```python
from build123d import *

# Parameters (mm, degrees)
F1_DEPTH = 5
F3_DEPTH = 2
F4_R     = 3.5
F5_DEPTH = 5
F6_R     = 2
F7_DEPTH = 5000


with BuildPart() as f1:
    # F0 (on Front) → F1 (new body)
    with BuildSketch(Plane.XZ):
        with BuildLine():
            Line((19.9153833091, -4.2498749681), (11.3317733631, 0))
            Line((11.3317733631, 0), (9.8158549517, -3.3205298241))
            Line((9.8158549517, -3.3205298241), (12.4476579949, -2.8994414024))
            Line((12.4476579949, -2.8994414024), (16.0058550537, -4.4364142232))
            add(Edge.make_bspline(
                [(16.0058550537, -4.4364142232), (20.2167406678, -7.2366520762), (14.6583728492, -14.2898829654), (8.973678574, -6.310257595)],
                knots=[0, 0, 0, 0, 7.2775541924, 7.2775541924, 7.2775541924, 7.2775541924], degree=3))
            Line((8.973678574, -6.310257595), (7.3524885811, -9.7631821409))
            Line((7.3524885811, -9.7631821409), (6.3418764621, -14.3951550126))
            Line((6.3418764621, -14.3951550126), (6.1102770269, -19.4692704827))
            Line((6.1102770269, -19.4692704827), (8.973678574, -17.8059712052))
            Line((8.973678574, -17.8059712052), (12.5318756327, -18.0796794593))
            Line((12.5318756327, -18.0796794593), (14.805752784, -19.9956316501))
            Line((14.805752784, -19.9956316501), (15.7110933214, -23.7643718719))
            Line((15.7110933214, -23.7643718719), (12.7424206585, -28.4173991531))
            Line((12.7424206585, -28.4173991531), (6.8050744012, -34.1863110662))
            Line((6.8050744012, -34.1863110662), (0, -38.9025583863))
            Line((0, -38.9025583863), (2.3386615794, -39.8540049791))
            Line((2.3386615794, -39.8540049791), (6.8705515005, -36.8744730949))
            Line((6.8705515005, -36.8744730949), (16.5853220969, -32.5428880751))
            Line((16.5853220969, -32.5428880751), (21.242402494, -29.1627496481))
            Line((21.242402494, -29.1627496481), (24.5724655688, -25.9829144925))
            Line((24.5724655688, -25.9829144925), (27.7022235096, -20.8000354469))
            Line((27.7022235096, -20.8000354469), (30.9822093695, -14.7157851607))
            Line((30.9822093695, -14.7157851607), (33.3608239889, -9.8333628848))
            Line((33.3608239889, -9.8333628848), (34.0869277716, -5.7521588169))
            Line((34.0869277716, -5.7521588169), (36.115013063, -4.5252935961))
            Line((36.115013063, -4.5252935961), (36.7910414934, -2.7976669371))
            Line((36.7910414934, -2.7976669371), (31.8084657192, -4.7506359406))
            Line((31.8084657192, -4.7506359406), (27.0011555403, -5.2764355205))
            Line((27.0011555403, -5.2764355205), (19.9153833091, -4.2498749681))
        make_face()
    extrude(amount=F1_DEPTH)

    # F2 (on face) → F3 (join)
    with BuildSketch(Plane.XZ.offset(5)):
        with BuildLine():
            Line((21.7291433364, -9.4480654225), (19.2754138261, -13.0034713075))
            Line((19.2754138261, -13.0034713075), (22.6067081094, -10.5641065165))
            Line((22.6067081094, -10.5641065165), (24.4384426624, -9.6377115697))
            Line((24.4384426624, -9.6377115697), (25.5543254316, -10.2482894436))
            Line((25.5543254316, -10.2482894436), (25.1121837646, -11.7642078549))
            Line((25.1121837646, -11.7642078549), (23.5962662846, -13.0064180121))
            Line((23.5962662846, -13.0064180121), (22.8383075446, -14.3960108981))
            add(Edge.make_bspline(
                [(21.911913529, -16.1435268819), (27.8071500361, -24.3758074939), (31.3442908227, -12.5221665949), (22.8383075446, -14.3960108981)],
                knots=[0, 0, 0, 0, 1.9778821972, 1.9778821972, 1.9778821972, 1.9778821972], degree=3))
            Line((21.911913529, -16.1435268819), (21.7645317316, -19.7438336909))
            Line((21.7645317316, -19.7438336909), (21.1032004239, -21.6240121639))
            Line((21.1032004239, -21.6240121639), (19.9749078602, -20.8000354469))
            Line((19.9749078602, -20.8000354469), (19.3432737142, -18.4805691242))
            Line((19.3432737142, -18.4805691242), (18.669532612, -14.9644799531))
            Line((18.669532612, -14.9644799531), (17.7220832556, -18.7542755157))
            Line((17.7220832556, -18.7542755157), (17.9957915097, -21.5755682439))
            Line((17.9957915097, -21.5755682439), (19.0064031631, -25.0916555524))
            Line((19.0064031631, -25.0916555524), (21.3110515224, -29.0971975582))
            Line((21.3110515224, -29.0971975582), (21.0065729916, -25.6180167198))
            Line((21.0065729916, -25.6180167198), (22.227730602, -22.9441039264))
            Line((22.227730602, -22.9441039264), (24.7753150761, -20.6281188875))
            Line((24.7753150761, -20.6281188875), (27.7164391152, -20.7736660335))
            Line((27.7164391152, -20.7736660335), (29.8788421939, -16.7624897322))
            Line((29.8788421939, -16.7624897322), (29.1153732687, -16.1833055317))
            Line((29.1153732687, -16.1833055317), (27.7132410556, -13.6544601992))
            Line((27.7132410556, -13.6544601992), (27.4127833545, -10.1992078125))
            Line((27.4127833545, -10.1992078125), (28.2366167336, -7.8957052901))
            Line((28.2366167336, -7.8957052901), (30.3422380239, -6.2431930564))
            Line((30.3422380239, -6.2431930564), (26.4112614095, -6.5937256441))
            Line((26.4112614095, -6.5937256441), (23.707151413, -7.8957052901))
            Line((23.707151413, -7.8957052901), (21.7291433364, -9.4480654225))
        make_face()
        Polygon((30.567580834, -17.2849819064), (29.8788421939, -16.7624897322), (27.7164391152, -20.7736660335), (28.2492954284, -20.8000354469), (29.7553811609, -21.899909378), (30.0746022613, -21.6493815286), (29.0152207017, -19.7387114167), (30.9822093695, -20.3396249563), (31.3804323032, -19.7688815121), (30.2170477808, -18.2865038514), (32.2701707482, -17.6605526358), align=None)
    extrude(amount=F3_DEPTH)

    # F4 (on Front) → F5 (join)
    with BuildSketch(Plane.XZ):
        with Locations((23.4437491745, -2.6102589909)):
            Circle(F4_R)
    extrude(amount=F5_DEPTH)

    # F6 (on face) → F7 (cut)
    with BuildSketch(Plane.XZ.offset(5)):
        with Locations((23.4437491745, -2.6102589909)):
            Circle(F6_R)
    extrude(amount=-F7_DEPTH, mode=Mode.SUBTRACT)


solid = f1.part
```
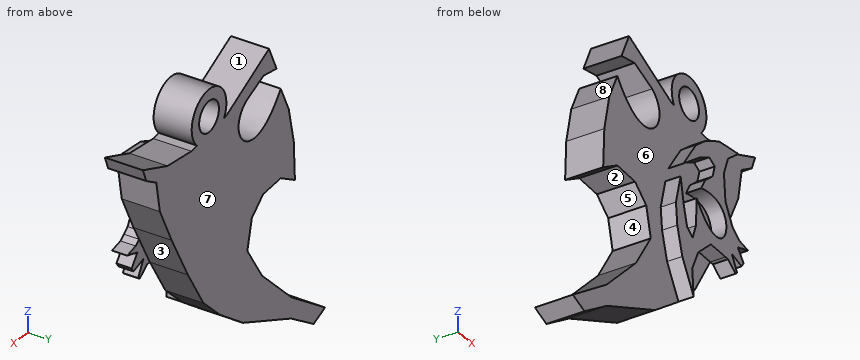
Model file for the job. Use its own axes, mm. Face numbers are marked on the shaded views. A direction names the side the tool comes from. Round coordinates to 2 decimals unless told otherwise and drop trailing zeros. Loops run counter-clockwise (first coordinate to the right, second up) from the corner with the lowest first, then second, coordinate; pieces in that order, holes last. Notation, with made-up numbers: M 10.5,-39.75 L 37.5,-39.75 A22 ccw 37.5,-23.75 Z; hole C -25.5,28 d8. An arc over 180 degrees is marked long. Put each result on its own line as item: value. Start each with the question number.
Item 1: Cut at C-C (z = -31). List the corners of the cut face in (x, y), then the cut area to 3 significant figures.
Item 2: Cut at B-B (x = 3.5). List the corners of the cut face in (y, z), then the cut area to 3 significant figures.
Item 3: Cut at A-A (z = -2). List the corners of the cut face in (x, y), then the cut area to 3 significant figures.
Item 4: Mould opens along Z. For the marked faces 5, 6, 7 and 8 say: released by +Z, released by -Z, zero draft, split by the parting line, or undercut.
Item 5: Drill centre lines: line 1 along Z through (x, y) = (11.5, -3.75); line 2 along X through (y, z) = (-2.25, -2.5); line 3 along Y through (x, z) = (29, -15). Where is each one in solid material? Low to high.
Item 6: Drop flat-ended pins along their axis: P1, Ø1.4, axis at x = 31, z = -18.5, coming from the +Y side; P2, Ø1.5, axis at x = 18.5, y = -2, coming from the +Z side; P3, Ø4, axis at y = -1, z = -12.5, coming from the +X side. Give the stop position or say it passes through.
Item 7: 3-axis set-ups, long thin cutter, end or side, ignore diameter. For the marked faces 1, 2, 3 and 4: which of +Z, -Z, +X, -X, +Y, -Y reach the whole face in a straight line?
Answer block:
1. outline: M 10.08,-5 L 18.71,-5 L 18.71,0 L 10.08,0 Z
1. area: 43.1 mm2
2. outline: M -5,-39.09 L 0,-39.09 L 0,-36.48 L -5,-36.48 Z
2. area: 13.1 mm2
3. outline: M 10.42,-5 L 15.37,-5 L 15.37,0 L 10.42,0 Z; M 20,-5 L 21.54,-5 L 21.54,0 L 20,0 Z; M 25.35,-5 L 26.89,-5 L 26.89,0 L 25.35,0 Z
3. area: 40.2 mm2
4. face 5: undercut
4. face 6: undercut
4. face 7: zero draft
4. face 8: released by +Z
5. line 1: -34.81 to -29.62, -18 to -8.96, -3.05 to -0.08
5. line 2: 10.19 to 16.38, 19.95 to 21.45, 25.44 to 26.94
5. line 3: -5 to 0
6. P1: y = -5
6. P2: z = -3.18
6. P3: x = 33.04
7. face 1: +Z, +Y, -Y
7. face 2: +Y, -Y
7. face 3: -Z, +X, +Y
7. face 4: -X, +Y, -Y
